```python
from build123d import *

# Parameters (mm, degrees)
F2_R     = 2
F4_DEPTH = 20


with BuildPart() as f1:
    # F0 (on Top) → F1 (revolve)
    with BuildSketch(Plane.XY):
        with BuildLine():
            Line((-8.75, 0), (0, 0))
            Line((0, 0), (0, 37))
            Line((0, 37), (-1.5, 37))
            Line((-1.5, 37), (-1.5, 15.3282299509))
            ThreePointArc((-1.5, 15.3282299509), (-4.3322917664, 13.3172311391), (-7.1645835327, 15.3282299509))
            Line((-7.1645835327, 15.3282299509), (-7.8059027445, 17.1648335314))
            ThreePointArc((-7.8059027445, 17.1648335314), (-8.2779513723, 17.5), (-8.75, 17.1648335314))
            Line((-8.75, 17.1648335314), (-8.75, 0))
        make_face()
    revolve(axis=Axis((0, 18.5, 0), (0, -1, 0)))

    # F2
    f2_edges = [f1.edges().sort_by_distance(p)[0] for p in [
        (1.5, 15.32823, 0),
    ]]
    fillet(f2_edges, radius=F2_R)

    # F3 (on face) → F4 (join)
    with BuildSketch(Plane.XZ):
        with BuildLine():
            Line((9.5e-09, 8.75), (-25, 8.75))
            Line((-25, 8.75), (-25, -8.75))
            Line((-25, -8.75), (0, -8.75))
            ThreePointArc((0, -8.75), (-8.75, 4.8e-09), (9.5e-09, 8.75))
        make_face()
        with BuildLine():
            Line((25, 8.75), (9.5e-09, 8.75))
            ThreePointArc((9.5e-09, 8.75), (6.1871843388, 6.187184332), (8.75, 0))
            ThreePointArc((8.75, 0), (6.1871843354, -6.1871843354), (0, -8.75))
            Line((0, -8.75), (25, -8.75))
            Line((25, -8.75), (25, 8.75))
        make_face()
        with BuildLine():
            ThreePointArc((8.75, 0), (6.1871843388, 6.187184332), (9.5e-09, 8.75))
            ThreePointArc((9.5e-09, 8.75), (-8.75, 4.8e-09), (0, -8.75))
            ThreePointArc((0, -8.75), (6.1871843354, -6.1871843354), (8.75, 0))
        make_face()
    extrude(amount=F4_DEPTH)


solid = f1.part
```
The listing builds one solid part. Answer for the finished solid, in the listing's coordinates (mm). A direction names the side the tool comes from. Give positions to 0.01 mm unless a question says otherwise; leave off trailing zeros. Order: outer loops, then holes, each group sorted by start corner. A loop starts at its lowest first (then second) coordinate and runs counter-clockwise, first axis right, second up. Notation, with made-up numbers: (80, 2.25) -> (96, 2.25) arc R4 cw to (96, 6.25) -> close; hole circle Ø5 at (82.25, 72). An arc over 180 degrees is marked (long way). One line per item, written item: value.
1) Find the intervals of material crossed by line 1 (X direction, y = 15, z = 1.25); line 2 (Y direction, x = -11.5, z = 3.75); line 3 (X direction, y = 3, z = 0), in increasing order.
Reported:
line 1: x = -8.66 to -6.92, -1.08 to 1.08, 6.92 to 8.66
line 2: y = -20 to 0
line 3: x = -8.75 to 8.75
2) Flat-ended cylindrical pins translate along their axes: P1, Ø8, axis at x = -12, y = 9, coming from the -Z side; P2, Ø5, axis at y = 17.5, z = -5, coming from the -X side; P3, Ø5, axis at y = 14, z = -0.5, coming from the +X side. Find the tip coordinate at first contact, or state that the pin passes through.
Reported:
P1: stops at z = -3.54
P2: stops at x = -8.38
P3: stops at x = 8.75
3) Find section A-A, the plane x = 20.5. Determine the outline of the cut face in (y, z), plus the area to 3 significant figures.
Reported:
outline: (-20, -8.75) -> (0, -8.75) -> (0, 8.75) -> (-20, 8.75) -> close
area: 350 mm^2
4) A tool of negligible diameter and unlimited length cuts with its end or side. For faces 1 (the cylindrical face through (6.944, 8.462, 5.324)), 2 (the flat face through (-25, -10, 0)), from which of +Z, -Z, +X, -X, +Y, -Y can it reach the whole face along a straight path? Write none if from no direction.
Reported:
face 1: +Y
face 2: +Z, -Z, -X, +Y, -Y
